Part model, mm, in its own coordinate system. A direction names the side the tool comes from. Give positions to 0.01 mm unless a question says otherwise; leave off trailing zeros. Write each loop counter-clockwise with the first axis right and the second up, starting at its lowest first coordinate (ties: lowest second). Pieces come first, ordered by that corner, then holes. Notation, with made-up numbers: M -22,16 L 30,16 A6 cw 30,22 Z; hole C -8,18.5 d5. An arc over 180 degrees is marked long. Use a Markdown table: item, result.
```python
from build123d import *

# Parameters (mm, degrees)
F0_W     = 120
F0_H     = 80
F1_DEPTH = 2
F3_DEPTH = 12
F4_R     = 2.5
F4_R_2   = 1
F5_DEPTH = 4
F6_W     = 8
F6_H     = 7
F6_W_2   = 10
F7_DEPTH = 3
F8_R     = 1


with BuildPart() as f1:
    # F0 (on Top) → F1 (new body)
    with BuildSketch(Plane.XY):
        Rectangle(F0_W, F0_H)
    extrude(amount=F1_DEPTH)

    # F2 (on face) → F3 (join)
    with BuildSketch(Plane.XY.offset(2)):
        with BuildLine():
            Line((-58, -34.1715728753), (-58, 34.1715728753))
            ThreePointArc((-58, 34.1715728753), (-59.4494897428, 35.2679491924), (-60, 37))
            Line((-60, 37), (-60, -37))
            ThreePointArc((-60, -37), (-59.4494897428, -35.2679491924), (-58, -34.1715728753))
        make_face()
        with BuildLine():
            ThreePointArc((-57, -40), (-59.1213203436, -39.1213203436), (-60, -37))
            Line((-60, -37), (-60, -40))
            Line((-60, -40), (-57, -40))
        make_face()
        with BuildLine():
            ThreePointArc((-57, -40), (-55.2679491924, -39.4494897428), (-54.1715728753, -38))
            Line((-54.1715728753, -38), (-55.7510004003, -38))
            ThreePointArc((-55.7510004003, -38), (-58.1313708499, -38.1313708499), (-58, -35.7510004003))
            Line((-58, -35.7510004003), (-58, -34.1715728753))
            ThreePointArc((-58, -34.1715728753), (-59.4494897428, -35.2679491924), (-60, -37))
            ThreePointArc((-60, -37), (-59.1213203436, -39.1213203436), (-57, -40))
        make_face()
        with BuildLine():
            Line((-55.7510004003, -38), (-54.1715728753, -38))
            ThreePointArc((-54.1715728753, -38), (-54.043204321, -37.5073059362), (-54, -37))
            ThreePointArc((-54, -37), (-55.2679491924, -34.5505102572), (-58, -34.1715728753))
            Line((-58, -34.1715728753), (-58, -35.7510004003))
            ThreePointArc((-58, -35.7510004003), (-56.307179677, -35.5577794898), (-55.4, -37))
            ThreePointArc((-55.4, -37), (-55.4902981487, -37.5299059542), (-55.7510004003, -38))
        make_face()
        with BuildLine():
            ThreePointArc((57, -40), (55.2679491924, -39.4494897428), (54.1715728753, -38))
            Line((54.1715728753, -38), (-54.1715728753, -38))
            ThreePointArc((-54.1715728753, -38), (-55.2679491924, -39.4494897428), (-57, -40))
            Line((-57, -40), (57, -40))
        make_face()
        with BuildLine():
            Line((58, -35.7510004003), (58, -34.1715728753))
            ThreePointArc((58, -34.1715728753), (54.8786796564, -34.8786796564), (54.1715728753, -38))
            Line((54.1715728753, -38), (55.7510004003, -38))
            ThreePointArc((55.7510004003, -38), (55.8686291501, -35.8686291501), (58, -35.7510004003))
        make_face()
        with BuildLine():
            ThreePointArc((60, -37), (59.4494897428, -35.2679491924), (58, -34.1715728753))
            Line((58, -34.1715728753), (58, -35.7510004003))
            ThreePointArc((58, -35.7510004003), (58.4422205102, -36.307179677), (58.6, -37))
            ThreePointArc((58.6, -37), (57.5299059542, -38.5097018513), (55.7510004003, -38))
            Line((55.7510004003, -38), (54.1715728753, -38))
            ThreePointArc((54.1715728753, -38), (55.2679491924, -39.4494897428), (57, -40))
            ThreePointArc((57, -40), (59.1213203436, -39.1213203436), (60, -37))
        make_face()
        with BuildLine():
            Line((60, -40), (60, -37))
            ThreePointArc((60, -37), (59.1213203436, -39.1213203436), (57, -40))
            Line((57, -40), (60, -40))
        make_face()
        with BuildLine():
            ThreePointArc((60, 37), (59.4494897428, 35.2679491924), (58, 34.1715728753))
            Line((58, 34.1715728753), (58, -34.1715728753))
            ThreePointArc((58, -34.1715728753), (59.4494897428, -35.2679491924), (60, -37))
            Line((60, -37), (60, 37))
        make_face()
        with BuildLine():
            ThreePointArc((58, 35.7510004003), (55.8686291501, 35.8686291501), (55.7510004003, 38))
            Line((55.7510004003, 38), (54.1715728753, 38))
            ThreePointArc((54.1715728753, 38), (54.8786796564, 34.8786796564), (58, 34.1715728753))
            Line((58, 34.1715728753), (58, 35.7510004003))
        make_face()
        with BuildLine():
            Line((-54.1715728753, 38), (54.1715728753, 38))
            ThreePointArc((54.1715728753, 38), (55.2679491924, 39.4494897428), (57, 40))
            Line((57, 40), (-57, 40))
            ThreePointArc((-57, 40), (-55.2679491924, 39.4494897428), (-54.1715728753, 38))
        make_face()
        with BuildLine():
            Line((54.1715728753, 38), (55.7510004003, 38))
            ThreePointArc((55.7510004003, 38), (57.5299059542, 38.5097018513), (58.6, 37))
            ThreePointArc((58.6, 37), (58.4422205102, 36.307179677), (58, 35.7510004003))
            Line((58, 35.7510004003), (58, 34.1715728753))
            ThreePointArc((58, 34.1715728753), (59.4494897428, 35.2679491924), (60, 37))
            ThreePointArc((60, 37), (59.1213203436, 39.1213203436), (57, 40))
            ThreePointArc((57, 40), (55.2679491924, 39.4494897428), (54.1715728753, 38))
        make_face()
        with BuildLine():
            Line((60, 40), (57, 40))
            ThreePointArc((57, 40), (59.1213203436, 39.1213203436), (60, 37))
            Line((60, 37), (60, 40))
        make_face()
        with BuildLine():
            ThreePointArc((-60, 37), (-59.1213203436, 39.1213203436), (-57, 40))
            Line((-57, 40), (-60, 40))
            Line((-60, 40), (-60, 37))
        make_face()
        with BuildLine():
            Line((-55.7510004003, 38), (-54.1715728753, 38))
            ThreePointArc((-54.1715728753, 38), (-55.2679491924, 39.4494897428), (-57, 40))
            ThreePointArc((-57, 40), (-59.1213203436, 39.1213203436), (-60, 37))
            ThreePointArc((-60, 37), (-59.4494897428, 35.2679491924), (-58, 34.1715728753))
            Line((-58, 34.1715728753), (-58, 35.7510004003))
            ThreePointArc((-58, 35.7510004003), (-58.1313708499, 38.1313708499), (-55.7510004003, 38))
        make_face()
        with BuildLine():
            ThreePointArc((-54, 37), (-54.043204321, 37.5073059362), (-54.1715728753, 38))
            Line((-54.1715728753, 38), (-55.7510004003, 38))
            ThreePointArc((-55.7510004003, 38), (-55.4902981487, 37.5299059542), (-55.4, 37))
            ThreePointArc((-55.4, 37), (-56.307179677, 35.5577794898), (-58, 35.7510004003))
            Line((-58, 35.7510004003), (-58, 34.1715728753))
            ThreePointArc((-58, 34.1715728753), (-55.2679491924, 34.5505102572), (-54, 37))
        make_face()
    extrude(amount=F3_DEPTH)

    # F4 (on face) → F5 (join)
    with BuildSketch(Plane.XY.offset(2)):
        with Locations((50, -25)):
            Circle(F4_R)
        with Locations((50, -25)):
            Circle(F4_R_2, mode=Mode.SUBTRACT)
        with Locations((1.6, -24)):
            Circle(F4_R)
        with Locations((1.6, -24)):
            Circle(F4_R_2, mode=Mode.SUBTRACT)
        with Locations((44.8, 27.2)):
            Circle(F4_R)
        with Locations((44.8, 27.2)):
            Circle(F4_R_2, mode=Mode.SUBTRACT)
        with Locations((16.8, 27.2)):
            Circle(F4_R)
        with Locations((16.8, 27.2)):
            Circle(F4_R_2, mode=Mode.SUBTRACT)
        with Locations((-48, 32)):
            Circle(F4_R)
        with Locations((-48, 32)):
            Circle(F4_R_2, mode=Mode.SUBTRACT)
        with Locations((-8, 32)):
            Circle(F4_R)
        with Locations((-8, 32)):
            Circle(F4_R_2, mode=Mode.SUBTRACT)
        with Locations((-8, -32)):
            Circle(F4_R)
        with Locations((-8, -32)):
            Circle(F4_R_2, mode=Mode.SUBTRACT)
        with Locations((-48, -32)):
            Circle(F4_R)
        with Locations((-48, -32)):
            Circle(F4_R_2, mode=Mode.SUBTRACT)
    extrude(amount=F5_DEPTH)

    # F6 (on face) → F7 (cut)
    with BuildSketch(Plane.XZ.offset(40)):
        with Locations((14.2, 10.5)):
            Rectangle(F6_W, F6_H)
        with Locations((44.2, 10.5)):
            Rectangle(F6_W_2, F6_H)
    extrude(amount=-F7_DEPTH, mode=Mode.SUBTRACT)

    # F8
    f8_edges = [f1.edges().sort_by_distance(p)[0] for p in [
        (60, -40, 7),
        (60, 40, 7),
        (-60, -40, 7),
        (-60, 40, 7),
    ]]
    fillet(f8_edges, radius=F8_R)


solid = f1.part
```
1. Drop flat-ended pins along their axis: P1, Ø0.6, axis at x = 16.5, y = 27.5, coming from the +Z side; P2, Ø23, axis at x = 4.5, y = -19, coming from the +Z side; P3, Ø0.6, axis at y = -39.5, z = 11.5, coming from the +X side. Give the stop position or say it passes through.
Findings below:
| item | result |
|---|---|
| P1 | z = 2 |
| P2 | z = 6 |
| P3 | x = 59.98 |
2. Cut at C-C, the plane z = 11. Give the cut face in (x, y), then the cut area to 3 significant figures.
Findings below:
| item | result |
|---|---|
| outline | M -60,-39 A1 ccw -59,-40 L 10.2,-40 L 10.2,-38 L -54.17,-38 A3 ccw -58,-34.17 L -58,34.17 A3 ccw -54.17,38 L 54.17,38 A3 ccw 58,34.17 L 58,-34.17 A3 ccw 54.17,-38 L 49.2,-38 L 49.2,-40 L 59,-40 A1 ccw 60,-39 L 60,39 A1 ccw 59,40 L -59,40 A1 ccw -60,39 Z; M 18.2,-40 L 39.2,-40 L 39.2,-38 L 18.2,-38 Z; hole C -57,-37 d3.2; hole C -57,37 d3.2; hole C 57,-37 d3.2; hole C 57,37 d3.2 |
| area | 771 mm2 |
3. Tool access for faces 1 (the flat face through (-1, 1, 0)), 2 (the cylindrical face through (16.26, 24.76, 3.97)): list every direction of +Z, -Z, +X, -X, +Y, -Y with a clear straight run to the whole face (end or side of a thin tool).
Findings below:
| item | result |
|---|---|
| face 1 | -Z, +X, -X, +Y, -Y |
| face 2 | +Z |
4. Cut at D-D, the plane x = -40. Give the cut face in (y, z), then the cut area to 3 significant figures.
Findings below:
| item | result |
|---|---|
| outline | M -40,0 L 40,0 L 40,14 L 38,14 L 38,2 L -38,2 L -38,14 L -40,14 Z |
| area | 208 mm2 |
5. Two-plate mould, pull along X, no slides. Class faces 3 (the cylindrical face through (-8.33, -29.52, 3.97)), 4 (the flat face through (-27, 39, 14)), 5 (the flat face through (60, -1, 7)): released by +X, released by -X, zero draft, split by the parting line, or undercut.
Findings below:
| item | result |
|---|---|
| face 3 | undercut |
| face 4 | zero draft |
| face 5 | released by +X |
6. Cut at A-A, the plane z = 4. State how many separate pieces and enclosed holes the cut face has, then the cut area to 3 significant figures.
Findings below:
| item | result |
|---|---|
| separate pieces | 9 |
| enclosed holes | 13 |
| area | 939 mm2 |
7. Drill centre lines: L1, parallel to Y at x = -57, z = 9; L2, parallel to Y at x = 50, z = 5.75; L3, parallel to X at y = -37, z = 10. Where is each one in solid material? Low to high.
Findings below:
| item | result |
|---|---|
| L1 | -40 to -38.6, -35.4 to -34, 34 to 35.4, 38.6 to 40 |
| L2 | -40 to -38, -27.5 to -26, -24 to -22.5, 38 to 40 |
| L3 | -60 to -58.6, -55.4 to -54, 54 to 55.4, 58.6 to 60 |
8. Cut at B-B, the plane y = 21. Give the cut face in (x, z), then the cut area to 3 significant figures.
Findings below:
| item | result |
|---|---|
| outline | M -60,0 L 60,0 L 60,14 L 58,14 L 58,2 L -58,2 L -58,14 L -60,14 Z |
| area | 288 mm2 |
